Autodesk Inventor part; units mm, degrees
ref_plane "YZ Plane" through (0, 0, 0) normal (1, 0, 0) x (0, 1, 0)
ref_plane "XZ Plane" through (0, 0, 0) normal (0, 1, 0) x (-1, 0, 0)
ref_plane "XY Plane" through (0, 0, 0) normal (0, 0, 1) x (1, 0, 0)
sketch "Sketch1" plane through (0, 0, 0) normal (0, 1, 0) x (-1, 0, 0)
  line L0 (3.1776, 14.7647) -> (24.1776, 14.7647)
  line L1 (24.1776, 14.7647) -> (24.1776, -15.2353)
  line L2 (24.1776, -15.2353) -> (3.1776, -15.2353)
  line L3 (3.1776, -15.2353) -> (3.1776, 14.7647)
  dimension "d4" = 30
  dimension "d5" = 21
extrude "Extrusion1" add sketch "Sketch1" along normal blind 91
fillet "Fillet1" radius 10 2 edges at (-3.1776, 45.5, 14.7647) (-24.1776, 45.5, 14.7647)
fillet "Fillet2" radius 6 2 edges at (-13.6776, 91, -15.2353) (-13.6776, 0, -15.2353)
sketch "Sketch2" plane through (0, 91, 0) normal (0, 1, 0) x (1, 0, 0)
  line L0 (-3.1776, 15.2353) -> (-3.1776, 7.2353)
  line L1 (-24.1776, 7.2353) -> (-24.1776, 15.2353)
  line L2 (-9.1776, 15.2353) -> (-3.1776, 15.2353)
  line L3 (-3.1776, 15.2353) -> (-3.1776, 7.2353)
  line L4 (-3.1776, 7.2353) -> (1.8224, 7.2353) construction
  arc A0 (-3.1776, 7.2353) -> (-9.1776, 15.2353) centre (-11.5109, 7.2353) ccw
  line L5 (-24.1776, 15.2353) -> (-18.1776, 15.2353)
  line L6 (-24.1776, 7.2353) -> (-24.1776, 15.2353)
  arc A1 (-18.1776, 15.2353) -> (-24.1776, 7.2353) centre (-15.8442, 7.2353) ccw
  line L7 (-24.1776, 15.2353) -> (-18.1776, 15.2353)
  line L8 (-3.1776, 15.2353) -> (-9.1776, 15.2353)
  point P0 (0, 0)
  dimension "d10" = 21
  dimension "d11" = 8
  dimension "d12" = 6
  dimension "d20" = 8
  dimension "d21" = 6
extrude "Extrusion3" cut sketch "Sketch2" against normal up to next
sketch "Sketch3" plane through (0, 91, 0) normal (0, 1, 0) x (1, 0, 0)
  line L0 (-9.1776, -6.2647) -> (-15.1776, -6.2647)
  line L1 (-15.1776, -6.2647) -> (-15.1776, 5.7353)
  line L2 (-15.1776, 5.7353) -> (-9.1776, 5.7353)
  line L3 (-9.1776, 5.7353) -> (-9.1776, -6.2647)
  line L4 (-3.1776, -4.7647) -> (-3.1776, 7.2353)
  line L5 (-14.1776, -14.7647) -> (-13.1776, -14.7647)
  point P0 (0, 0)
  dimension "d24" = 6
  dimension "d25" = 12
  dimension "d26" = 6
  dimension "d27" = 8.5
sketch "Sketch4" plane through (0, 91, 0) normal (0, 1, 0) x (1, 0, 0)
  line L0 (-9.6776, -5.7647) -> (-11.6776, -5.7647)
  line L1 (-11.6776, -5.7647) -> (-11.6776, 5.2353)
  line L2 (-11.6776, 5.2353) -> (-9.6776, 5.2353)
  line L3 (-9.6776, 5.2353) -> (-9.6776, -5.7647)
  line L4 (-3.1776, -4.7647) -> (-3.1776, 7.2353)
  line L5 (-14.1776, -14.7647) -> (-13.1776, -14.7647)
  point P0 (0, 0)
  dimension "d28" = 2
  dimension "d29" = 11
  dimension "d30" = 6.5
  dimension "d31" = 9
extrude "Extrusion4" cut sketch "Sketch3" against normal blind 10
extrude "Extrusion5" add sketch "Sketch4" against normal blind 10
sketch "Sketch5" plane through (0, 91, 0) normal (0, 1, 0) x (1, 0, 0)
  arc A0 (-13.1776, -14.7647) -> (-3.1776, -4.7647) centre (-13.1776, -4.7647) ccw
  line L0 (-14.1776, -14.7647) -> (-13.1776, -14.7647)
  arc A1 (-24.1776, -4.7647) -> (-14.1776, -14.7647) centre (-14.1776, -4.7647) ccw
  line L1 (-24.1776, 7.2353) -> (-24.1776, -4.7647)
  arc A2 (-23.934, 9.2353) -> (-24.1776, 7.2353) centre (-15.8442, 7.2353) ccw
  line L2 (-9.1776, 15.2353) -> (-18.1776, 15.2353)
  arc A3 (-3.1776, 7.2353) -> (-3.4211, 9.2353) centre (-11.5109, 7.2353) ccw
  line L3 (-3.1776, -4.7647) -> (-3.1776, 7.2353)
  line L4 (-9.1776, -6.2647) -> (-15.1776, -6.2647)
  line L5 (-9.1776, 5.7353) -> (-9.1776, -6.2647)
  line L6 (-15.1776, 5.7353) -> (-9.1776, 5.7353)
  line L7 (-15.1776, -6.2647) -> (-15.1776, 5.7353)
  point P0 (0, 0)
properties part number "Powerbank"
The listing builds one solid part. Answer for the finished solid, in the listing's coordinates (mm). A direction names the side the tool comes from. Coordinates: 2 decimals unless noted, no trailing zeros. Loops run counter-clockwise (first coordinate to the right, second up) from the corner with the lowest first, then second, coordinate; pieces in that order, holes last. Notation, with made-up numbers: (32, -13.5) -> (65, -13.5) arc R17 ccw to (65, 15.5) -> close; hole circle Ø4 at (1, -5). An arc over 180 degrees is marked (long way). Write item = value, one per line. Start each with the question number.
1) The mould has two halves that part along Z. Classify faces 1 (the face through (-9.178, 86, 0)), 2 (the face through (-24.178, 45, -1)), 3 (the face through (-14, 45, -15.235)), 4 (the face through (-9.678, 86, 0)): released by +Z, released by -Z, zero draft, split by the parting line, or undercut.
2) A cutting plane is placed at A-A (z = -2). Give the vertices of the cut face in (x, y).
3) Straight lines are drawn through the part: line 1 (Z direction, x = -16, y = 15); line 2 (Z direction, x = -7, y = 34.5); line 3 (X direction, y = 45, z = 9.5). For each, find the intervals that lie inside material, in ascending order. Write a range as from..to.
4) A cutting plane is placed at B-B (y = 63.5). Give the vertices of the cut face in (x, z), then the cut area to 3 significant figures.
5) A tool of negligible diameter and unlimited length cuts with its end or side. For faces 5 (the face through (-11, 86, -5.235)), 6 (the face through (-21.326, 46.137, 11.758)), from which of +Z, -Z, +X, -X, +Y, -Y can it reach the whole face along a straight path? Write none if from no direction.
6) A cutting plane is placed at C-C (x = -10.75). Give the vertices of the cut face in (y, z), then the cut area to 3 significant figures.
7) Given pin 1 Ø5 at (x, z) = (-12, 0) entering from +Y; pin 2 Ø2 at (x, y) = (-10, 86) entering from +Z; pin 3 Ø2 at (y, z) = (30, 11.5) entering from +X; pin 4 Ø3 at (x, y) = (-11, 85) entering from +Z, each flat-ended and moving along its own axis, determine where each tip first touches the part or whether it passes through.
8) A cutting plane is placed at D-D (x = -19.5). Give the vertices of the cut face in (y, z).
Responses:
q1.face_1 = undercut
q1.face_2 = zero draft
q1.face_3 = released by -Z
q1.face_4 = undercut
q2.outline = (-24.18, 0) -> (-3.18, 0) -> (-3.18, 91) -> (-9.18, 91) -> (-9.18, 81) -> (-9.68, 81) -> (-9.68, 91) -> (-11.68, 91) -> (-11.68, 81) -> (-15.18, 81) -> (-15.18, 91) -> (-24.18, 91) -> close
q3.line_1 = -15.24..14.6
q3.line_2 = -14.24..12.63
q3.line_3 = -22.99..-4.37
q4.outline = (-24.18, -7.24) arc R8.33 ccw to (-18.18, -15.24) -> (-9.18, -15.24) arc R8.33 ccw to (-3.18, -7.24) -> (-3.18, 4.76) arc R10 ccw to (-13.18, 14.76) -> (-14.18, 14.76) arc R10 ccw to (-24.18, 4.76) -> close
q4.area = 562 mm²
q5.face_5 = +Y
q5.face_6 = +Z, -X, +Y, -Y
q6.outline = (0, -9.24) arc R6 ccw to (6, -15.24) -> (85, -15.24) arc R6 ccw to (91, -9.24) -> (91, -5.74) -> (81, -5.74) -> (81, -5.24) -> (91, -5.24) -> (91, 5.76) -> (81, 5.76) -> (81, 6.26) -> (91, 6.26) -> (91, 14.47) -> (0, 14.47) -> close
q6.area = 2,680 mm²
q7.pin_1 = 91
q7.pin_2 = 14.52
q7.pin_3 = -4.99
q7.pin_4 = 14.74
q8.outline = (0, -9.24) arc R6 ccw to (3.58, -14.72) -> (87.42, -14.72) arc R6 ccw to (91, -9.24) -> (91, 13.23) -> (0, 13.23) -> close
